Autodesk Fusion 360 part; units mm, degrees
sketch "Sketch1" plane through (0, 0, 0) normal (0, 0, 1) x (1, 0, 0)
  line L0 (0, 19) -> (0, 75)
  line L1 (0, 75) -> (8, 75)
  line L2 (10, 68) -> (10, 24)
  line L3 (24, 10) -> (160, 10)
  line L4 (10, 68) -> (8, 68)
  line L5 (8, 68) -> (8, 75)
  arc A0 (0, 19) -> (19, 0) centre (19, 19) ccw
  arc A1 (10, 24) -> (24, 10) centre (24, 24) ccw
  circle A2 centre (152.5, 2.5) radius 3.175
  circle A3 centre (152.5, 2.5) radius 5
  line L6 (160, -5) -> (148.2812, -5)
  line L7 (148.2812, -5) -> (138, 0)
  line L8 (19, 0) -> (138, 0)
  line L9 (160, 10) -> (160, -5)
  line L10 (24, 10) -> (24, 0)
  point P0 (10, 10)
  dimension "d1" = 7
  dimension "d2" = 75
  dimension "d5" = 19
  dimension "d6" = 14
  dimension "d13" = 6.35
  dimension "d14" = 10
  dimension "d18" = 7.5
  dimension "d19" = 15
  dimension "d20" = 119
  dimension "d42" = 7.5
  dimension "d43" = 160
extrude "Extrude1" add sketch "Sketch1" along normal blind 20 contours L0 L1 L2 L4 L5 A0 A1 L8 L10 | L3 L6 L7 L8 L9 L10 | A3
extrude "Extrude3" cut sketch "Sketch1" along normal blind 15 contours A3
sketch "Sketch2" plane through (0, 0, 0) normal (-1, 0, 0) x (0, -1, 0)
  line L0 (-75, 0) -> (-19, 0)
  line L1 (-19, 0) -> (-19, 20)
  line L2 (-19, 20) -> (-75, 20)
  line L3 (-75, 20) -> (-75, 0)
  circle A0 centre (-65, 10) radius 2.6
  circle A1 centre (-65, 10) radius 5
  line L4 (-68, 20) -> (-68, 0)
  line L5 (-62, 20) -> (-62, 0)
  dimension "d23" = 5.2
  dimension "d24" = 10
  dimension "d25" = 10
  dimension "d26" = 10
  dimension "d31" = 20
  dimension "d32" = 20
  dimension "d33" = 7
  dimension "d34" = 13
extrude "Extrude4" cut sketch "Sketch2" against normal blind 10 contours A0
extrude "Extrude5" cut sketch "Sketch2" against normal blind 7 contours A1 L4 L5 | A1 L4 | A1 L5
extrude "Extrude6" add sketch "Sketch2" against normal blind 1 from surface at -10 contours L0 A1 L4 L5 | A1 L4 L5 | L2 A1 L4 L5
sketch "Sketch5" plane through (0, 10, 0) normal (0, 1, 0) x (-1, 0, 0)
  line L0 (-160, 0) -> (-24, 0)
  line L1 (-24, 0) -> (-24, 20)
  line L2 (-24, 20) -> (-160, 20)
  line L3 (-160, 20) -> (-160, 0)
  line L4 (-24, 0) -> (-160, 10)
extrude "Extrude8" cut sketch "Sketch5" against normal blind 15 contours L0 L3 L4
equation "d20 = 69 mm + 50 mm"
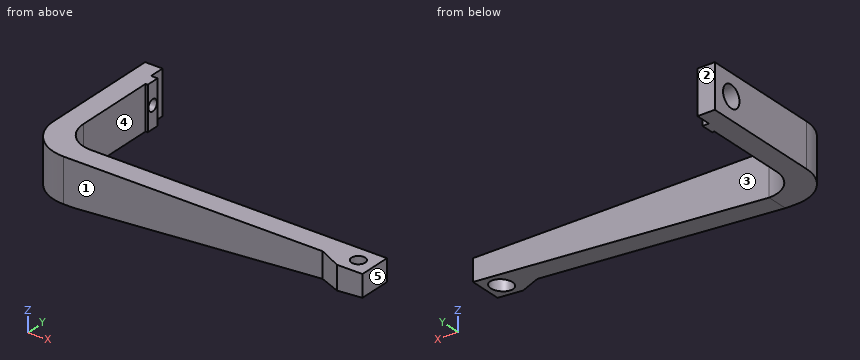
Work out the finished part from the listing and answer in its coordinate system (mm). Face numbers are marked on the shaded views. A direction names the side the tool comes from. Coordinates: 2 decimals unless noted, no trailing zeros. Write each loop counter-clockwise with the first axis right and the second up, starting at its lowest first coordinate (ties: lowest second). Pieces come first, ordered by that corner, then holes.
Q1. A cutting plane is placed at D-D, the plane y = 42. Give the vertices of the cut face in (x, z), then the cut area to 3 significant figures.
Q2. Find the intervals of material crossed by line 1 (Z direction, x = 4, y = 65); line 2 (Y direction, x = 152.5, z = 18.75) (3 decimals); line 3 (Y direction, x = 152.5, z = 10.4), in increasing order.
Q3. A cutting plane is placed at A-A, the plane y = 65. Give the vertices of the cut face in (x, z).
Q4. A cutting plane is placed at B-B, the plane z = 17. Give the vertices of the cut face in (x, y) (3 decimals), then the cut area to 3 significant figures.
Q5. Each of these flat-tipped pins is pushed along its axis until it touches: pin 1 Ø3 at (y, z) = (64.5, 12) entering from -X; pin 2 Ø10 at (x, z) = (60.5, 11) entering from +Y; pin 3 Ø7.5 at (x, y) = (152.5, 2.5) entering from -Z. Where does it stop, or does it pass through?
Q6. Which of the six approach directions +Z, -Z, +X, -X, +Y, -Y give full straight-line access (tool end or side, diameter ignored) to the marked faces 1 and 2?
Q7. A cutting plane is placed at C-C, the plane x = 152.5. Give the vertices of the cut face in (y, z) (3 decimals), then the cut area to 3 significant figures.
Q8. Determine the mould class of the marked faces 3, 4 and 5 for opening direction Y: released by +Y, released by -Y, zero draft, split by the parting line, or undercut.
Findings below:
1. outline: (0, 0) - (10, 0) - (10, 20) - (0, 20) - close
1. area: 200 mm2
2. line 1: z = 0 to 5, 15 to 20
2. line 2: y = -5 to -0.675, 5.675 to 10
2. line 3: y = -5 to -2.5, 7.5 to 10
3. outline: (0, 0) - (11, 0) - (11, 7.4) - (7, 7.4) - (7, 5) - (0, 5) - close; (0, 15) - (7, 15) - (7, 12.6) - (11, 12.6) - (11, 20) - (0, 20) - close
4. outline: (0, 19) arc R19 ccw to (19, 0) - (138, 0) - (148.281, -5) - (160, -5) - (160, 10) - (24, 10) arc R14 cw to (10, 24) - (10, 62) - (11, 62) - (11, 68) - (8, 68) - (8, 75) - (0, 75) - close; hole circle Ø6.35 at (152.5, 2.5)
4. area: 2,260 mm2
5. pin 1: stops at x = 7
5. pin 2: stops at y = 10
5. pin 3: stops at z = 15
6. face 1: +Z, -Z, -X, -Y
6. face 2: +Z, -Z, +X, -X, +Y
7. outline: (-5, 9.449) - (-2.5, 9.449) - (-2.5, 15) - (-0.675, 15) - (-0.675, 20) - (-5, 20) - close; (5.675, 15) - (7.5, 15) - (7.5, 9.449) - (10, 9.449) - (10, 20) - (5.675, 20) - close
7. area: 71.0 mm2
8. face 3: released by +Y
8. face 4: undercut
8. face 5: zero draft
